Build history of the part. All positions in model axes, mm. A direction names the side the tool comes from. Give positions to 0.01 mm unless a question says otherwise; leave off trailing zeros. Order: outer loops, then holes, each group sorted by start corner. A loop starts at its lowest first (then second) coordinate and runs counter-clockwise, first axis right, second up. Notation, with made-up numbers: (-2.75, -13.5) - (51.25, -13.5) arc R25 cw to (51.25, 0.5) - close; hole circle Ø3 at (68, 3.25). An arc over 180 degrees is marked (long way). Use a Markdown table: item, result. Add a question column.
(1) Mould opens along Y. For faces 4 (the face through (-4.06, -0.9, -2.11)), 5 (the face through (0, 0, -2.108)), 6 (the face through (-3.15, 2.41, -15.77)) say: +Y half, -Y half, draft (parallel to the pull), parting line (faces both ways), or undercut.
(2) Slice it at A-A (z = -21.5). Write the cut outline in (x, y).
(3) Flat gauge pins, fed straight in: pin 1 (4 mm diameter, centred on x = 0, y = -1, fed in from +Z); pin 2 (2 mm diameter, centred on x = -0.5, z = -4, fed in from -Y); pin 3 (0.8 mm diameter, centred on x = -0.5, z = 0.5, fed in from -Y); pin 4 (8 mm diameter, centred on x = -5.5, z = -21, fed in from -Y). Where does each tip first touch, or does it go through?
(4) Which spindle directions (+Z, -Z, +X, -X, +Y, -Y) get a long thin tool onto all of the face, cutting with end or side? Do faces 1 (the face through (3.874, -0.86, -2.891)), 2 (the face through (0, 0, -27.508)), 3 (the face through (2.072, 1.174, -0.199)). Say none if no direction does.
(5) Wall check: line 1 (Z direction, x = 5, y = 1.5); line 2 (Y direction, x = -0.75, z = -2); line 3 (Y direction, x = -3.25, z = -7). Give the ranges that are in metal, low to high.
Solid Edge part; units mm, degrees
sketch "Sketch1" plane through (0, 0, 0) normal (1, 0, 0) x (0, 1, 0)
  line L0 (0, -2.1082) -> (0, 2.1082)
  arc A0 (0, 2.1082) -> (6.9469, -2.1082) centre (-0.3606, -6.3169) cw
  line L1 (0, -2.1082) -> (6.9469, -2.1082)
revolve "RevolvedProtrusion1" add sketch "Sketch1" angle 360 about axis through (0, 0, -14.7796) along (0, 0, 1)
sketch "Sketch2" plane through (0, 0, -2.1082) normal (0, 0, -1) x (0, 1, 0)
  circle A0 centre (0, 0) radius 3.9687
extrude "Protrusion1" add sketch "Sketch2" along normal blind 25.4
sketch "Sketch3" plane through (0, 0, -27.5082) normal (0, 0, -1) x (1, 0, 0)
  circle A0 centre (0, 0) radius 3.9662
extrude "Cutout1" cut sketch "Sketch3" against normal blind 23.8125 flip side to cut
sketch "Sketch4" plane through (-0.6032, 0.3606, 4.2164) normal (0, 0, 1) x (1, 0, 0)
  line L0 (-0.7716, 2.0206) -> (1.978, 2.0206)
  line L1 (3.3529, -0.3606) -> (1.978, 2.0206)
  line L2 (1.978, -2.7419) -> (3.3529, -0.3606)
  line L3 (-0.7716, -2.7419) -> (1.978, -2.7419)
  line L4 (-2.1464, -0.3606) -> (-0.7716, -2.7419)
  line L5 (-0.7716, 2.0206) -> (-2.1464, -0.3606)
extrude "ExtrudedCutout_11" cut sketch "Sketch4" against normal blind 6.3246
properties part number "146368"
Solution:
| question | item | result |
|---|---|---|
| 1 | face 4 | draft |
| 1 | face 5 | undercut |
| 1 | face 6 | parting line |
| 2 | outline | circle Ø7.93 at (0, 0) |
| 3 | pin 1 | z = 1.66 |
| 3 | pin 2 | y = -3.97 |
| 3 | pin 3 | y = -5.09 |
| 3 | pin 4 | y = -3.67 |
| 4 | face 1 | -Z |
| 4 | face 2 | -Z, +X, -X, +Y, -Y |
| 4 | face 3 | +Z |
| 5 | line 1 | -2.11 to 0.01 |
| 5 | line 2 | -6.84 to -2.38, 2.38 to 6.84 |
| 5 | line 3 | -2.27 to 2.27 |
